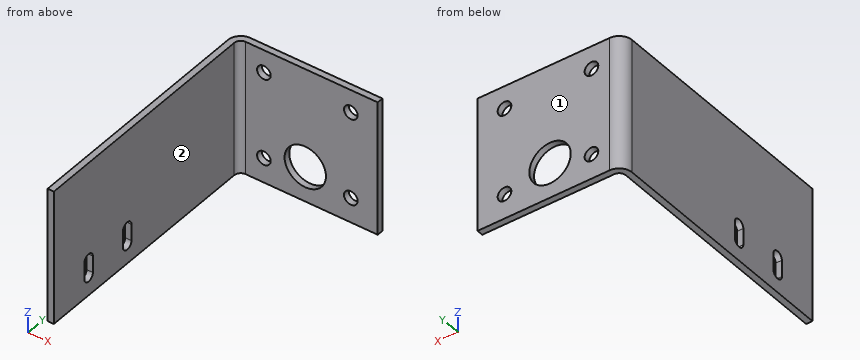
```python
from build123d import *

# Parameters (mm, degrees)
SKETCH1_W                    = 70
SKETCH1_H                    = 65
BASE_FLANGE1_DEPTH           = 3.03784
EDGE_FLANGE1_STRIP_W         = 18.50136
EDGE_FLANGE1_STRIP_H         = 3.03784
EDGE_FLANGE1_STRIP_CUT_DEPTH = 65
EDGE_FLANGE1_DEPTH           = 65
CUT_EXTRUDE1_DEPTH           = 146.239664251
M6_CLEARANCE_HOLE1_D         = 6.6
SKETCH12_R                   = 10
CUT_EXTRUDE2_DEPTH           = 3.03784


# Sheet-metal steps are written as plain solids
with BuildPart() as part:
    # Sketch1 → Base-Flange1 (new body)
    with BuildSketch(Plane(origin=(0, 0, 0), x_dir=(1, 0, 0), z_dir=(0, 1, 0))):
        with Locations((35, 0)):
            Rectangle(SKETCH1_W, SKETCH1_H)
    extrude(amount=-BASE_FLANGE1_DEPTH)

    # Edge-Flange1 strip (across the edge) → Edge-Flange1 strip cut (cut)
    with BuildSketch(Plane(origin=(0, -3.03784, 32.5), x_dir=(1, 0, 0), z_dir=(0, 0, -1))):
        with Locations((-3.03784, -1.51892)):
            Rectangle(EDGE_FLANGE1_STRIP_W, EDGE_FLANGE1_STRIP_H)
    extrude(amount=EDGE_FLANGE1_STRIP_CUT_DEPTH, mode=Mode.SUBTRACT)

    # Edge-Flange1 section (across the edge) → Edge-Flange1 (add)
    with BuildSketch(Plane(origin=(0, -3.03784, 32.5), x_dir=(1, 0, 0), z_dir=(0, 0, -1))):
        with BuildLine():
            Line((0, 3.175), (0, 120))
            Line((0, 120), (3.03784, 120))
            Line((3.03784, 120), (3.03784, 3.175))
            ThreePointArc((3.03784, 3.175), (3.96777597, 0.92993597), (6.21284, 0))
            Line((6.21284, 0), (6.21284, -3.03784))
            ThreePointArc((6.21284, -3.03784), (1.819698706, -1.218141294), (0, 3.175))
        make_face()
    extrude(amount=EDGE_FLANGE1_DEPTH)

    # Sketch9 → Cut-Extrude1 (cut, through all)
    with BuildSketch(Plane.ZY):
        with BuildLine():
            Line((-23, -72.75), (-15, -72.75))
            ThreePointArc((-15, -72.75), (-12.25, -75.5), (-15, -78.25))
            Line((-15, -78.25), (-23, -78.25))
            ThreePointArc((-23, -78.25), (-25.75, -75.5), (-23, -72.75))
        make_face()
        with BuildLine():
            Line((-23, -97.75), (-15, -97.75))
            ThreePointArc((-15, -97.75), (-12.25, -100.5), (-15, -103.25))
            Line((-15, -103.25), (-23, -103.25))
            ThreePointArc((-23, -103.25), (-25.75, -100.5), (-23, -97.75))
        make_face()
    extrude(amount=-CUT_EXTRUDE1_DEPTH, mode=Mode.SUBTRACT)

    # M6 Clearance Hole1 (through all)
    with Locations(Plane(origin=(0, 0, 0), x_dir=(1, 0, 0), z_dir=(0, 1, 0))):
        with Locations((57, 20.5), (57, -21.5), (15, -21.5), (15, 20.5)):
            Hole(M6_CLEARANCE_HOLE1_D / 2)

    # Sketch12 → Cut-Extrude2 (cut)
    with BuildSketch(Plane.XZ.offset(3.03784)):
        with Locations(Location((35, -15.5, 0), (0, 0, 270))):
            Circle(SKETCH12_R)
    extrude(amount=-CUT_EXTRUDE2_DEPTH, mode=Mode.SUBTRACT)


solid = part.part
```
Geometry: final body of the model. Coordinates: model frame, mm. Face numbers are marked on the shaded views. A direction names the side the tool comes from. Round coordinates to 2 decimals unless told otherwise and drop trailing zeros. Loops run counter-clockwise (first coordinate to the right, second up) from the corner with the lowest first, then second, coordinate; pieces in that order, holes last. Notation, with made-up numbers: (7.5, -18.75) -> (48.5, -18.75) arc R11 cw to (48.5, -13.75) -> close; hole circle Ø8 at (-4, 17.25). An arc over 180 degrees is marked (long way). Write each question's results on one line, items separated by ' | '.
Item 1: Set-up query: the marked faces 1 and 2. Return all of +Z, -Z, +X, -X, +Y, -Y with unobstructed straight access to the full face (end or side cutting, diameter ignored); none if empty.
Answers below:
face 1: +Z, -Z, +X, -X, +Y | face 2: +Z, -Z, +X, -Y
Item 2: Line query: probe 1 along X at (y, z) = (-1, 21); probe 2 along X at (y, z) = (-1.7, 21.5); probe 3 along X at (y, z) = (-1.9, -20.5). Output: solid intervals per line, ascending. Write a range as [from, to].
Answers below:
probe 1: x = [2.83, 11.74], [18.26, 53.74], [60.26, 70] | probe 2: x = [1.94, 11.7], [18.3, 53.7], [60.3, 70] | probe 3: x = [1.74, 11.7], [18.3, 26.34], [43.66, 53.7], [60.3, 70]
Item 3: Cut plane B-B on z = 21.5. Return the cut outline in (x, y) (3 decimals).
Answers below:
outline: (0, -123.038) -> (3.038, -123.038) -> (3.038, -6.213) arc R3.175 cw to (6.213, -3.038) -> (11.7, -3.038) -> (11.7, 0) -> (6.213, 0) arc R6.213 ccw to (0, -6.213) -> close; (18.3, -3.038) -> (53.7, -3.038) -> (53.7, 0) -> (18.3, 0) -> close; (60.3, -3.038) -> (70, -3.038) -> (70, 0) -> (60.3, 0) -> close
Item 4: Cut plane D-D on z = -9. Return the cut outline in (x, y) (3 decimals), and give its area (3 significant figures).
Answers below:
outline: (0, -123.038) -> (3.038, -123.038) -> (3.038, -6.213) arc R3.175 cw to (6.213, -3.038) -> (27.401, -3.038) -> (27.401, 0) -> (6.213, 0) arc R6.213 ccw to (0, -6.213) -> close; (42.599, -3.038) -> (70, -3.038) -> (70, 0) -> (42.599, 0) -> close | area: 525 mm²
Item 5: Cut plane C-C on y = -100.5. Return the cut outline in (x, z), and give its area (3 significant figures).
Answers below:
outline: (0, -32.5) -> (3.04, -32.5) -> (3.04, -25.75) -> (0, -25.75) -> close; (0, -12.25) -> (3.04, -12.25) -> (3.04, 32.5) -> (0, 32.5) -> close | area: 156 mm²
Item 6: Cut plane A-A on x = 35. Return the cut outline in (y, z), and give its area (3 significant figures).
Answers below:
outline: (-3.04, -32.5) -> (0, -32.5) -> (0, -25.5) -> (-3.04, -25.5) -> close; (-3.04, -5.5) -> (0, -5.5) -> (0, 32.5) -> (-3.04, 32.5) -> close | area: 137 mm²
Item 7: Pin query (flat end, axial travel): pin 1 Ø8.5 at (x, z) = (15, -20.5) entering from +Y; pin 2 Ø5.5 at (x, z) = (57, 21.5) entering from -Y; pin 3 Ø4 at (x, z) = (18, -10) entering from -Y; pin 4 Ø1.5 at (x, z) = (2.5, -18) entering from +Y. Return the tip coordinate at first contact, or that it passes through.
Answers below:
pin 1: stops at y = 0 | pin 2: passes through | pin 3: stops at y = -3.04 | pin 4: stops at y = -0.75
